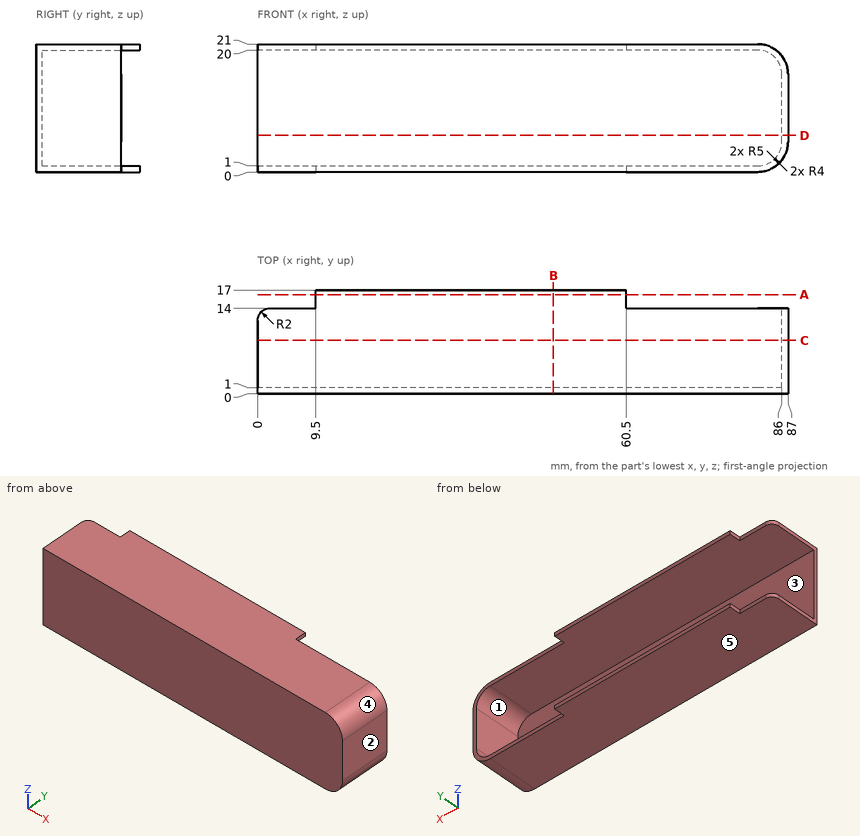
Can you work these out from the drawing? Everything is in mm from the part's minimum corner. A direction names the side the tool comes from. Give positions to 0.01 mm unless a question says otherwise; leave off trailing zeros. Order: outer loops, then holes, each group sorted by start corner. A loop starts at its lowest first (then second) coordinate and runs counter-clockwise, first axis right, second up.
Item 1: I'm going to push flat-ended pins straight in: pin 1 (0.8 mm diameter, centred on y = 15, z = 0.5, fed in from -X); pin 2 (0.5 mm diameter, centred on x = 7, z = 20.5, fed in from +Y); pin 3 (3 mm diameter, centred on x = 58, z = 8, fed in from +Y). Where does each tip first touch, or does it pass through?
Item 2: For the marked faces 1 and 2, which set-ups out of +Z, -Z, +X, -X, +Y, -Y let a thin tool reach every point of the face, with its end or its side?
Item 3: If we mould it in two halves opening along Z, with no side actions, what happens to the marked faces 3, 4 and 5? For each: pulls with the +Z half, pulls with the -Z half, needs draft (parallel to the pull), parting line crosses it, or undercut.
Item 4: If we section it at D-D, the plane z = 6: Write out the boundary of the cut face in (x, y).
Item 5: If we section it at B-B, the plane x = 48.5: Write out the boundary of the cut face in (y, z).
Item 6: If we section it at C-C, the plane y = 8.75: Write out the boundary of the cut face in (x, z).
Item 7: I need wall thicknesses on line 1 (Z direction, x = 44.5, y = 6); line 2 (Y direction, x = 39, z = 4.5); line 3 (X direction, y = 10.25, z = 12). Which ranges of each line are inside material? Lowest first, please.
Item 8: If we section it at A-A, the plane y = 16.25: Write out the boundary of the cut face in (x, z).
Values:
1. pin 1: stops at x = 9.5
1. pin 2: stops at y = 14
1. pin 3: stops at y = 1
2. face 1: -X, +Y
2. face 2: +Z, -Z, +X, +Y, -Y
3. face 3: undercut
3. face 4: pulls with the +Z half
3. face 5: pulls with the -Z half
4. outline: (0, 0) - (87, 0) - (87, 14) - (86, 14) - (86, 1) - (0, 1) - close
5. outline: (0, 0) - (17, 0) - (17, 1) - (1, 1) - (1, 20) - (17, 20) - (17, 21) - (0, 21) - close
6. outline: (0, 0) - (82, 0) arc R5 ccw to (87, 5) - (87, 16) arc R5 ccw to (82, 21) - (0, 21) - (0, 20) - (82, 20) arc R4 cw to (86, 16) - (86, 5) arc R4 cw to (82, 1) - (0, 1) - close
7. line 1: z = 0 to 1, 20 to 21
7. line 2: y = 0 to 1
7. line 3: x = 86 to 87
8. outline: (9.5, 0) - (60.5, 0) - (60.5, 1) - (9.5, 1) - close; (9.5, 20) - (60.5, 20) - (60.5, 21) - (9.5, 21) - close
